from build123d import *

# Parameters (mm, degrees)
F0_R      = 5
F2_DEPTH  = 3.175
F2_FACE_R = 5
F3_R      = 2.25
F5_R      = 1.5
F6_DEPTH  = 25.4


with BuildPart() as f2:
    # F0 (on Top) → F2 (new body)
    with BuildSketch(Plane.XY):
        Circle(F0_R)
    extrude(amount=F2_DEPTH)

    # F2_face (on face) → F4 section 0
    with BuildSketch(Plane.XY.offset(3.175)):
        Circle(F2_FACE_R)
    # F3 (on offset) → F4 section 1
    with BuildSketch(Plane.XY.offset(5.55625)):
        Circle(F3_R)
    loft()

    # F5 (on face) → F6 (cut)
    with BuildSketch(Plane.XY.offset(5.55625)):
        Circle(F5_R)
    extrude(amount=-F6_DEPTH, mode=Mode.SUBTRACT)


solid = f2.part
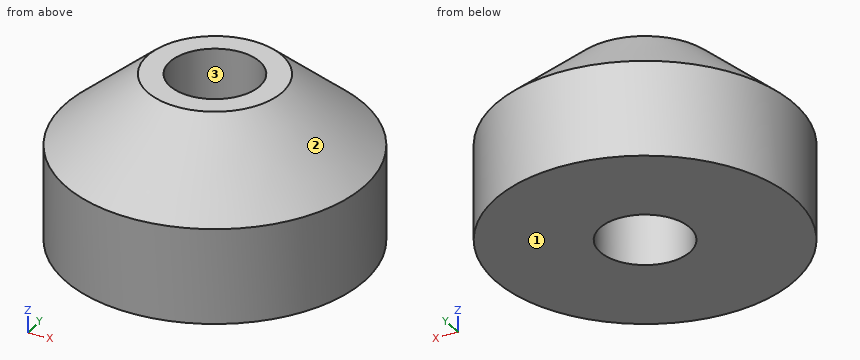
The model under review builds one solid part; all positions refer to its coordinate system, in mm. Face numbers are marked on the shaded views. Round coordinates to 2 decimals unless told otherwise and drop trailing zeros. Loops run counter-clockwise (first coordinate to the right, second up) from the corner with the lowest first, then second, coordinate; pieces in that order, holes last. Notation, with made-up numbers: M -34,-0.75 L -8,-0.75 A18 ccw -8,25.25 Z; hole C 33,76.5 d5. An arc over 180 degrees is marked long. Answer as a JSON object with one key per item and string values.
Item 1: The part is to be moulded in two halves that separate along Y. For the marked faces 1, 2 and 3, say which applies: +Y half, -Y half, draft (parallel to the pull), parting line (faces both ways), or undercut.
Check sheet entries:
{"face 1": "draft", "face 2": "parting line", "face 3": "undercut"}
Item 2: Clearance check with flat-ended pins moving along their axes: P1, Ø1, axis at x = -2, y = 2.5, coming from the +Z side; P2, Ø2, axis at y = -3.5, z = 3.5, coming from the -X side. State where each tip first meets the part, or that it passes through.
Check sheet entries:
{"P1": "z = 5.17", "P2": "x = -4.3"}
Item 3: We need section B-B, the plane z = 0.85. State the section outline as (x, y) points, and give its area (3 significant figures).
Check sheet entries:
{"outline": "C 0,0 d10; hole C 0,0 d3", "area": "71.5 mm2"}
Item 4: We need section A-A, the plane x = 0. State the section outline as (y, z) points (3 decimals).
Check sheet entries:
{"outline": "M -5,0 L -1.5,0 L -1.5,5.556 L -2.25,5.556 L -5,3.175 Z; M 1.5,0 L 5,0 L 5,3.175 L 2.25,5.556 L 1.5,5.556 Z"}
Item 5: We need section C-C, the plane z = 3.3. State the section outline as (x, y) points.
Check sheet entries:
{"outline": "C 0,0 d9.71; hole C 0,0 d3"}
Item 6: For line 1 along Y through (x, z) = (0, 3.15); line 2 along Y through (x, z) = (0, 4.3); line 3 along Z through (x, y) = (-4.25, -1.25), list the stretches that pass through material, from the lowest coordinate up.
Check sheet entries:
{"line 1": "-5 to -1.5, 1.5 to 5", "line 2": "-3.7 to -1.5, 1.5 to 3.7", "line 3": "0 to 3.67"}
